Could you check a few things on this drawing? It's one solid part, dimensions in mm from its lowest x, y, z. A direction names the side the tool comes from. Give positions to 0.01 mm unless a question says otherwise; leave off trailing zeros. Loops run counter-clockwise (first coordinate to the right, second up) from the corner with the lowest first, then second, coordinate; pieces in that order, holes last.
1. Imagine slicing it at B-B (z = 53.9). List the corners of the cut face in (x, y) for me, plus the area to 3 significant figures.
2. Thinking about a two-plate mould opening in X: for the marked faces 1, 2 and 3, which applies, +X half, -X half, draft (parallel to the pull), parting line (faces both ways), or undercut?
3. For the marked faces 4, 5, 6 and 7, which set-ups out of +Z, -Z, +X, -X, +Y, -Y let a thin tool reach every point of the face, with its end or its side?
4. For P1, Ø2, axis at x = 33, z = 52, coming from the +Y side; P2, Ø7.5, axis at y = 10.5, z = 53, coming from the +X side; P3, Ø3.5, axis at y = 20.1, z = 53.9, coming from the +X side; P4, Ø1.8, axis at y = 15, z = 20, coming from the +X side, each with a flat end and sliding along its axis, tell me the tip position at first contact or that it passes through.
5. I need wall thicknesses on line 1 along Z through (x, y) = (3.5, 15) (1 decimal); line 2 along Z through (x, y) = (28.35, 9.9); line 3 along X through (y, z) = (12, 43). Which ranges of each line are inside material? Lowest first, please.
6. Imagine slicing it at D-D (z = 20). List the corners of the cut face in (x, y) for me.
7. Imagine slicing it at A-A (y = 20.1). List the corners of the cut face in (x, z) for me.
8. Imagine slicing it at C-C (y = 15). Count the separate pieces of the cut face and the enclosed holes in it, plus the area to 3 significant figures.
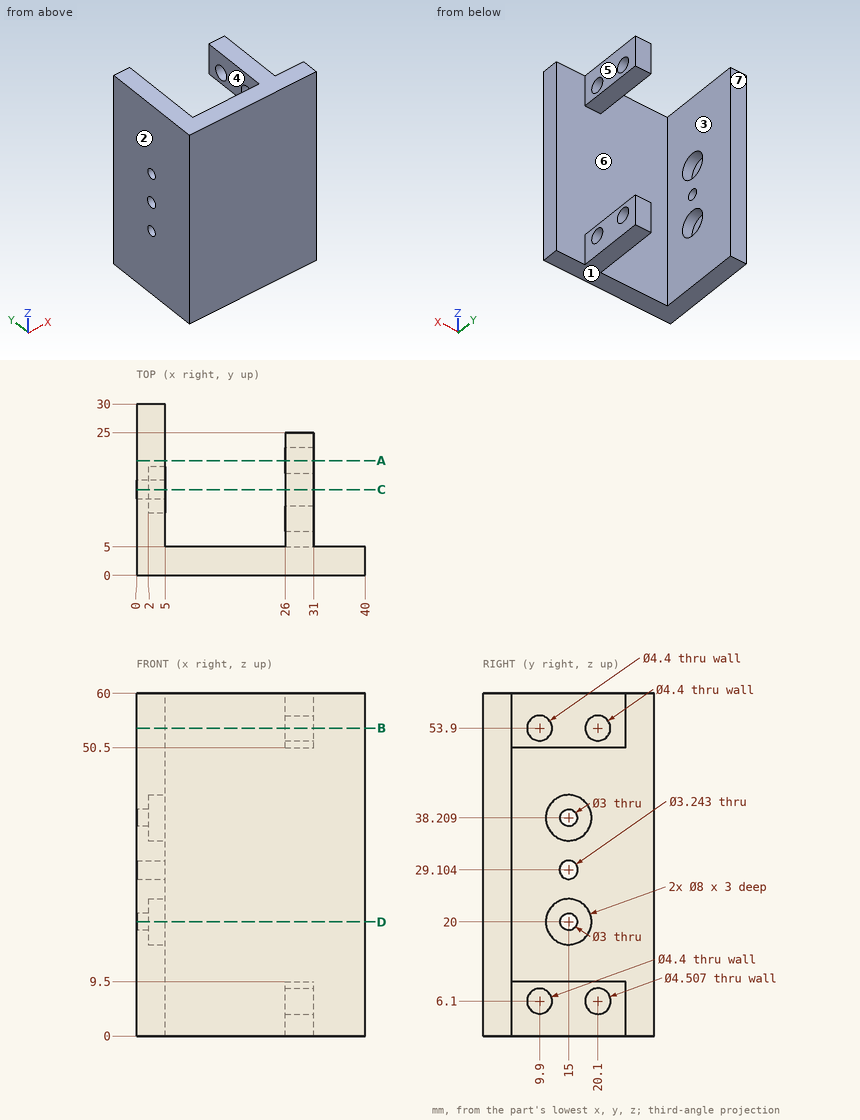
Derived:
1. outline: (0, 0) - (40, 0) - (40, 5) - (31, 5) - (31, 7.7) - (26, 7.7) - (26, 5) - (5, 5) - (5, 30) - (0, 30) - close; (26, 12.1) - (31, 12.1) - (31, 17.9) - (26, 17.9) - close; (26, 22.3) - (31, 22.3) - (31, 25) - (26, 25) - close
1. area: 381 mm2
2. face 1: draft
2. face 2: -X half
2. face 3: undercut
3. face 4: +Z, -Z, +Y
3. face 5: +Z, -Z, +X, +Y
3. face 6: +Y
3. face 7: +Z, -Z, +X, -X, +Y
4. P1: stops at y = 5
4. P2: stops at x = 31
4. P3: stops at x = 5
4. P4: passes through
5. line 1: z = 0 to 16, 24 to 27.5, 30.7 to 34.2, 42.2 to 60
5. line 2: z = 0 to 3.9, 8.3 to 9.5, 50.5 to 51.7, 56.1 to 60
5. line 3: x = 0 to 5
6. outline: (0, 0) - (40, 0) - (40, 5) - (5, 5) - (5, 11) - (2, 11) - (2, 13.5) - (0, 13.5) - close; (0, 16.5) - (2, 16.5) - (2, 19) - (5, 19) - (5, 30) - (0, 30) - close
7. outline: (0, 0) - (5, 0) - (5, 60) - (0, 60) - close; (26, 0) - (31, 0) - (31, 3.85) - (26, 3.85) - close; (26, 8.35) - (31, 8.35) - (31, 9.5) - (26, 9.5) - close; (26, 50.5) - (31, 50.5) - (31, 51.7) - (26, 51.7) - close; (26, 56.1) - (31, 56.1) - (31, 60) - (26, 60) - close
8. separate pieces: 6
8. enclosed holes: 0
8. area: 319 mm2
